Can you work these out from the model? Positions are in its coordinate system, mm. Face numbers are marked on the shaded views. Coordinates: 2 decimals unless noted, no trailing zeros. Order: outer loops, then holes, each group sorted by start corner. A loop starts at its lowest first (then second) coordinate and runs counter-clockwise, first axis right, second up. Notation, with made-up numbers: (11, -27.5) - (46, -27.5) arc R17 cw to (46, -16.5) - close; hole circle Ø1 at (-26, 20.5). An arc over 180 degrees is marked (long way). Return JSON: item names as keys, results as strings. Group by question number.
1) Imagine slicing it at A-A (y = 7.25). Write out the boundary of the cut face in (x, z), and give its area (3 significant figures).
2) Imagine slicing it at C-C (x = 26). Write out the boundary of the cut face in (y, z).
3) For pin 1 Ø4.5 at (x, z) = (36.08, 20.83) entering from +Y; pin 2 Ø4 at (x, y) = (2.5, 4.5) entering from +Z; pin 3 Ø4 at (x, y) = (8.5, 7.5) entering from +Z, each with a flat end and sliding along its axis, tell me the tip position at first contact or that it passes through.
4) If I drill on line 1 along X through (y, z) = (6, 0.5); line 2 along Y through (x, z) = (-34.5, 0); line 3 along X through (y, z) = (3.5, 0.5), over which ranges is the centre line in solid material (lowest first)?
5) Imagine slicing it at B-B (z = 25.5). Write out the boundary of the cut face in (x, y).
6) If we mould it in two halves opening along X, with no side actions, what happens to the marked faces 1 and 2? For each: pulls with the +X half, pulls with the -X half, needs draft (parallel to the pull), parting line crosses it, or undercut.
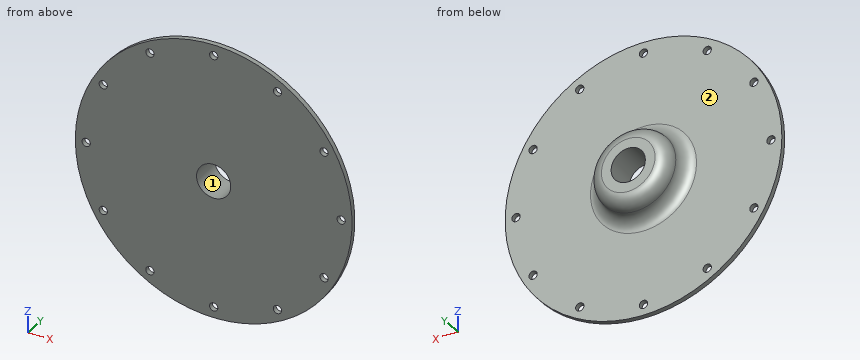
```python
from build123d import *

# Parameters (mm, degrees)
F_36_0_1065_DIAMETER_HOLE1_D = 2.7051
CIRPATTERN1_COUNT            = 12


with BuildPart() as part:
    # Sketch1 → Revolve1 (revolve)
    with BuildSketch(Plane.XY):
        with BuildLine():
            Line((-45.212, 0), (-5.588, 0))
            Line((-5.588, 0), (-5.588, 10.16))
            Line((-5.588, 10.16), (-8.763, 10.16))
            ThreePointArc((-8.763, 10.16), (-11.793836441, 8.904586441), (-13.04925, 5.87375))
            ThreePointArc((-13.04925, 5.87375), (-14.304663559, 2.842913559), (-17.3355, 1.5875))
            Line((-17.3355, 1.5875), (-45.212, 1.5875))
            Line((-45.212, 1.5875), (-45.212, 0))
        make_face()
    revolve(axis=Axis((0, 55, 0), (0, -1, 0)))

    # #36 (0.1065) Diameter Hole1 (through all)
    with Locations(Plane(origin=(0, 0, 0), x_dir=(-1, 0, 0), z_dir=(0, -1, 0))):
        with Locations((41.656, 0)):
            f_36_0_1065_diameter_hole1 = Hole(F_36_0_1065_DIAMETER_HOLE1_D / 2)

    # CirPattern1: #36 (0.1065) Diameter Hole1 ×12 about axis
    cirpattern1_axis = Axis((0, 0, 0), (0, 1, 0))
    for i in range(1, CIRPATTERN1_COUNT):
        add(f_36_0_1065_diameter_hole1.rotate(cirpattern1_axis, i * 360 / CIRPATTERN1_COUNT), mode=Mode.SUBTRACT)


solid = part.part
```
Calculated:
{
 "1": {"outline": "circle Ø25.64 at (0, 0); hole circle Ø11.18 at (0, 0)", "area": "418 mm2"},
 "2": {"outline": "(0, -36.99) - (1.59, -36.99) - (1.59, 36.99) - (0, 36.99) - close"},
 "3": {"pin 1": "y = 1.59", "pin 2": "z = 14.5", "pin 3": "z = 11.12"},
 "4": {"line 1": "-13.04 to -5.57, 5.57 to 13.04", "line 2": "0 to 1.59", "line 3": "-13.76 to -5.57, 5.57 to 13.76"},
 "5": {"outline": "(-37.33, 0) - (37.33, 0) - (37.33, 1.59) - (-37.33, 1.59) - close"},
 "6": {"face 1": "undercut", "face 2": "needs draft"}
}
